```python
from build123d import *

# Parameters (mm, degrees)
CROQUIS1_W              = 15
CROQUIS1_H              = 13
SALIENTE_EXTRUIR1_DEPTH = 1.2
CORTAR_EXTRUIR1_REACH   = 3.2
CROQUIS2_W              = 0.95
CROQUIS2_H              = 3.725
CORTAR_EXTRUIR2_REACH   = 3.2
CROQUIS3_R              = 4.2


with BuildPart() as part:
    # Croquis1 → Saliente-Extruir1 (new body)
    with BuildSketch(Plane.XY):
        Rectangle(CROQUIS1_W, CROQUIS1_H)
    extrude(amount=SALIENTE_EXTRUIR1_DEPTH)

    # Croquis2 → Cortar-Extruir1 (cut, up to next)
    with BuildSketch(Plane.XY.offset(1.2), mode=Mode.PRIVATE) as cortar_extruir1_sk1:
        with Locations((7.025, 4.6375)):
            Rectangle(CROQUIS2_W, CROQUIS2_H)
    cortar_extruir1_tool1 = extrude(cortar_extruir1_sk1.sketch, amount=-CORTAR_EXTRUIR1_REACH, mode=Mode.PRIVATE) & part.part
    add(cortar_extruir1_tool1.solids().sort_by_distance((7.025, 4.6375, 1.2))[0], mode=Mode.SUBTRACT)
    # Croquis2 → Cortar-Extruir1 (cut, up to next)
    with BuildSketch(Plane.XY.offset(1.2), mode=Mode.PRIVATE) as cortar_extruir1_sk2:
        with Locations((7.025, -4.6375)):
            Rectangle(CROQUIS2_W, CROQUIS2_H)
    cortar_extruir1_tool2 = extrude(cortar_extruir1_sk2.sketch, amount=-CORTAR_EXTRUIR1_REACH, mode=Mode.PRIVATE) & part.part
    add(cortar_extruir1_tool2.solids().sort_by_distance((7.025, -4.6375, 1.2))[0], mode=Mode.SUBTRACT)
    # Croquis2 → Cortar-Extruir1 (cut, up to next)
    with BuildSketch(Plane.XY.offset(1.2), mode=Mode.PRIVATE) as cortar_extruir1_sk3:
        with Locations((-7.025, -4.6375)):
            Rectangle(CROQUIS2_W, CROQUIS2_H)
    cortar_extruir1_tool3 = extrude(cortar_extruir1_sk3.sketch, amount=-CORTAR_EXTRUIR1_REACH, mode=Mode.PRIVATE) & part.part
    add(cortar_extruir1_tool3.solids().sort_by_distance((-7.025, -4.6375, 1.2))[0], mode=Mode.SUBTRACT)
    # Croquis2 → Cortar-Extruir1 (cut, up to next)
    with BuildSketch(Plane.XY.offset(1.2), mode=Mode.PRIVATE) as cortar_extruir1_sk4:
        with Locations((-7.025, 4.6375)):
            Rectangle(CROQUIS2_W, CROQUIS2_H)
    cortar_extruir1_tool4 = extrude(cortar_extruir1_sk4.sketch, amount=-CORTAR_EXTRUIR1_REACH, mode=Mode.PRIVATE) & part.part
    add(cortar_extruir1_tool4.solids().sort_by_distance((-7.025, 4.6375, 1.2))[0], mode=Mode.SUBTRACT)

    # Croquis3 → Cortar-Extruir2 (cut, up to next)
    with BuildSketch(Plane.XY.offset(1.2), mode=Mode.PRIVATE) as cortar_extruir2_sk1:
        Circle(CROQUIS3_R)
    cortar_extruir2_tool1 = extrude(cortar_extruir2_sk1.sketch, amount=-CORTAR_EXTRUIR2_REACH, mode=Mode.PRIVATE) & part.part
    add(cortar_extruir2_tool1.solids().sort_by_distance((0, 0, 1.2))[0], mode=Mode.SUBTRACT)


solid = part.part
```
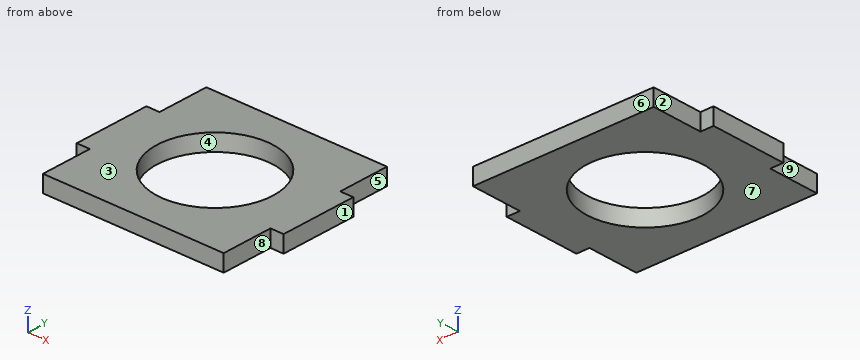
CAD build for the part. Positions are in the model's coordinates, mm. Face numbers are marked on the shaded views. A direction names the side the tool comes from. Round coordinates to 2 decimals unless told otherwise and drop trailing zeros. Loops run counter-clockwise (first coordinate to the right, second up) from the corner with the lowest first, then second, coordinate; pieces in that order, holes last. Notation, with made-up numbers: M -29.5,15 L 13.5,15 A16 cw 13.5,41 Z; hole C 6.25,60 d1. An arc over 180 degrees is marked long. Return JSON: item names as keys, results as strings. Group by question number.
(1) Saw through at C-C, the plane y = 0. List the corners of the cut face in (x, z), and give its area (3 significant figures).
(2) Saw through at D-D, the plane y = 5.5. List the corners of the cut face in (x, z), and give its area (3 significant figures).
(3) Mould opens along X. For the marked faces 1, 2, 3 and 4 say: +X half, -X half, draft (parallel to the pull), parting line (faces both ways), or undercut.
(4) Drop flat-ended pins along their axis: P1, Ø0.5, axis at x = -7, z = 0.5, coming from the +Y side (3 decimals); P2, Ø0.6, axis at y = -4, z = 0.5, coming from the +X side; P3, Ø6.5, axis at x = 0, y = 0, coming from the -Z side. Give the stop position or say it passes through.
(5) Saw through at A-A, the plane x = 0. List the corners of the cut face in (y, z), and give its area (3 significant figures).
(6) Saw through at B-B, the plane z = 0.5. List the corners of the cut face in (x, y) (3 decimals).
(7) Wall check: probe 1 along Y at (x, z) = (0, 0.3); probe 2 along X at (y, z) = (0.75, 0.9); probe 3 along X at (y, z) = (-3.75, 0.55). Give the ranges that are in metal, low to high. Write a range as [from, to].
(8) Tool access for the marked faces 5, 6, 7, 8 and 9: list every direction of +Z, -Z, +X, -X, +Y, -Y with a clear straight run to the whole face (end or side of a thin tool).
Answer list:
{
 "1": {"outline": "M -7.5,0 L -4.2,0 L -4.2,1.2 L -7.5,1.2 Z; M 4.2,0 L 7.5,0 L 7.5,1.2 L 4.2,1.2 Z", "area": "7.92 mm2"},
 "2": {"outline": "M -6.55,0 L 6.55,0 L 6.55,1.2 L -6.55,1.2 Z", "area": "15.7 mm2"},
 "3": {"face 1": "+X half", "face 2": "-X half", "face 3": "draft", "face 4": "undercut"},
 "4": {"P1": "y = 2.775", "P2": "x = 6.55", "P3": "through"},
 "5": {"outline": "M -6.5,0 L -4.2,0 L -4.2,1.2 L -6.5,1.2 Z; M 4.2,0 L 6.5,0 L 6.5,1.2 L 4.2,1.2 Z", "area": "5.52 mm2"},
 "6": {"outline": "M -7.5,-2.775 L -6.55,-2.775 L -6.55,-6.5 L 6.55,-6.5 L 6.55,-2.775 L 7.5,-2.775 L 7.5,2.775 L 6.55,2.775 L 6.55,6.5 L -6.55,6.5 L -6.55,2.775 L -7.5,2.775 Z; hole C 0,0 d8.4"},
 "7": {"probe 1": "[-6.5, -4.2], [4.2, 6.5]", "probe 2": "[-7.5, -4.13], [4.13, 7.5]", "probe 3": "[-6.55, -1.89], [1.89, 6.55]"},
 "8": {"face 5": "+Z, -Z, +X, +Y", "face 6": "+Z, -Z, +X, -X, +Y", "face 7": "-Z, +X, -X, +Y, -Y", "face 8": "+Z, -Z, +X, -Y", "face 9": "+Z, -Z, -X, -Y"}
}
